Verification items for the finished model (mm, model axes). A direction names the side the tool comes from. Give positions to 0.01 mm unless a question says otherwise; leave off trailing zeros. Order: outer loops, then holes, each group sorted by start corner. A loop starts at its lowest first (then second) coordinate and runs counter-clockwise, first axis right, second up.
from build123d import *

# Parameters (mm, degrees)
SKETCH1_R           = 2.7559
BOSS_EXTRUDE1_DEPTH = 3.7
BOSS_EXTRUDE2_START = 3.7
SKETCH1_3_R         = 2.7559
BOSS_EXTRUDE2_DEPTH = 2.3


with BuildPart() as part:
    # Sketch1 → Boss-Extrude1 (new body)
    with BuildSketch(Plane(origin=(0, 0, 0), x_dir=(1, 0, 0), z_dir=(0, 1, 0))):
        with Locations(Location((0, 0, 0), (0, 0, 270))):
            Circle(SKETCH1_R)
        Polygon((-2.05, -0.585), (-2.05, 0.585), (-0.585, 0.585), (-0.585, 2.05), (0.585, 2.05), (0.585, 0.585), (2.05, 0.585), (2.05, -0.585), (0.585, -0.585), (0.585, -2.05), (-0.585, -2.05), (-0.585, -0.585), align=None, mode=Mode.SUBTRACT)
    extrude(amount=BOSS_EXTRUDE1_DEPTH)

    # Sketch1<3> → Boss-Extrude2 (add)
    with BuildSketch(Plane(origin=(0, 0, 0), x_dir=(1, 0, 0), z_dir=(0, 1, 0)).offset(BOSS_EXTRUDE2_START)):
        with Locations(Location((0, 0, 0), (0, 0, 270))):
            Circle(SKETCH1_3_R)
    extrude(amount=BOSS_EXTRUDE2_DEPTH)


solid = part.part
(1) Go/stop test with flat-tipped pins: pin 1 (1.6 mm diameter, centred on x = -1, y = 2.5, fed in from +Z); pin 2 (2 mm diameter, centred on x = -1.5, y = 3.5, fed in from -Z); pin 3 (1.2 mm diameter, centred on y = 2.5, z = -1, fed in from -X). Record where each tip stops, or that it passes through.
Solved:
pin 1: stops at z = 2.75
pin 2: stops at z = -2.71
pin 3: stops at x = -2.73
(2) Set-up check for faces 5 (the flat face through (2.05, 2, 0)), 6 (the flat face through (0, 6, 0)): record each of +Z, -Z, +X, -X, +Y, -Y from which the full face is reachable in a straight line by a thin tool's end or side.
Solved:
face 5: -Y
face 6: +Z, -Z, +X, -X, +Y
(3) Section check A-A, the plane y = 3.6. Enter the section's corners in (x, z) (3 decimals).
Solved:
outline: circle Ø5.512 at (0, 0); hole (-2.05, -0.585) - (-0.585, -0.585) - (-0.585, -2.05) - (0.585, -2.05) - (0.585, -0.585) - (2.05, -0.585) - (2.05, 0.585) - (0.585, 0.585) - (0.585, 2.05) - (-0.585, 2.05) - (-0.585, 0.585) - (-2.05, 0.585) - close
(4) Section check B-B, the plane x = 0. Enter the section's corners in (y, z).
Solved:
outline: (0, -2.76) - (6, -2.76) - (6, 2.76) - (0, 2.76) - (0, 2.05) - (3.7, 2.05) - (3.7, -2.05) - (0, -2.05) - close
(5) Scan lines: line 1 (Z direction, x = -0.1, y = 1.65); line 2 (Z direction, x = 0.55, y = 1.1); line 3 (X direction, y = 3.2, z = -1.3) (3 decimals). Record each from-to range of solid material in increasing order.
Solved:
line 1: z = -2.75 to -2.05, 2.05 to 2.75
line 2: z = -2.7 to -2.05, 2.05 to 2.7
line 3: x = -2.43 to -0.585, 0.585 to 2.43
(6) Section check C-C, the plane z = 0. Enter the section's corners in (x, y), then the cut area to 3 significant figures.
Solved:
outline: (-2.76, 0) - (-2.05, 0) - (-2.05, 3.7) - (2.05, 3.7) - (2.05, 0) - (2.76, 0) - (2.76, 6) - (-2.76, 6) - close
area: 17.9 mm2
(7) Release check for a two-part mould opening along Z. For faces 1 (the flat face through (1, 0, -1)), 2 (the flat face through (0, 2, -2.05)), 3 (the flat face through (1, 2, -0.585)), 4 (the cylindrical face through (1.863, 2.958, -2.031)) record: pulls with the +Z half, pulls with the -Z half, needs draft (parallel to the pull), parting line crosses it, or undercut.
Solved:
face 1: needs draft
face 2: undercut
face 3: undercut
face 4: parting line crosses it
